Verification items for the finished model (mm, model axes). A direction names the side the tool comes from. Coordinates: 2 decimals unless noted, no trailing zeros. Order: outer loops, then holes, each group sorted by start corner. A loop starts at its lowest first (then second) coordinate and runs counter-clockwise, first axis right, second up.
Q1. Thickness scan on line 1 (X direction, y = 3, z = 6); line 2 (X direction, y = -8, z = 3.75); line 3 (X direction, y = -3, z = 0.5). Record the ranges inside material, lowest first.
Q2. Cross-section at D-D, the plane z = 1.25. Record the boundary of the cut face in (x, y), and give its area (3 significant figures).
Q3. Cross-section at B-B, the plane x = 0. Record the boundary of the cut face in (y, z) (3 decimals).
Q4. Depth check by flat-ended pin: P1, Ø10, axis at x = 2, y = -6, coming from the +Z side (3 decimals); P2, Ø1, axis at y = 10.5, z = 5.5, coming from the +X side; P3, Ø4.5, axis at x = -12.97, z = 4.76, coming from the +Y side; P4, Ø3, axis at x = -11.5, z = 4, coming from the +Y side. Enter the tip coordinate at first touch or a pass-through.
Q5. Draft check along Y on faces 1 (the flat face through (10, -12, 0)), 2 (the flat face through (26, 5.5, 7)), 3 (the flat face through (21, -1.5, 5)). Enter one of: pulls with the +Y half, pulls with the -Y half, needs draft (parallel to the pull), parting line crosses it, or undercut.
Q6. Cross-section at A-A, the plane y = -12.5. Record the boundary of the cut face in (x, z) (1 decimal), and give its area (3 significant figures).
Q7. Cross-section at C-C, the plane y = 10.5. Record the boundary of the cut face in (x, z) (3 decimals), and give its area (3 significant figures).
Q8. Set-up check for faces 4 (the flat face through (21, 1.5, 5)), 5 (the cylindrical face through (21.731, 3.472, 5.716)), 6 (the cylindrical face through (-14.572, -15.061, 5.991)): record each of +Z, -Z, +X, -X, +Y, -Y from which the full face is reachable in a straight line by a thin tool's end or side.
from build123d import *

# Parameters (mm, degrees)
BOSS_EXTRUDE1_DEPTH        = 9.525
F_10_CLEARANCE_HOLE1_D     = 4.9784
F_10_CLEARANCE_HOLE1_DEPTH = 4
F_10_CLEARANCE_HOLE1_TIP   = 1.495662253
F_10_32_TAPPED_HOLE1_D     = 4.0386
F_10_32_TAPPED_HOLE2_D     = 4.0386
F_10_32_TAPPED_HOLE2_DEPTH = 7
F_10_32_TAPPED_HOLE2_TIP   = 1.213317848


with BuildPart() as part:
    # Sketch1 → Boss-Extrude1 (new body)
    with BuildSketch(Plane.XY):
        with BuildLine():
            ThreePointArc((14.221111068, -1.5), (-14.3, 0), (14.221111068, 1.5))
            Line((14.221111068, 1.5), (28.530488985, 1.5))
            Line((28.530488985, 1.5), (28.530488985, 5.5))
            Line((28.530488985, 5.5), (19.530488985, 5.5))
            ThreePointArc((19.530488985, 5.5), (17.886036082, 5.990861772), (16.779715889, 7.302816901))
            ThreePointArc((16.779715889, 7.302816901), (-3.729691625, 17.915897979), (-18.3, 0))
            Line((-18.3, 0), (-18.3, -18.61))
            Line((-18.3, -18.61), (28.530488985, -18.61))
            Line((28.530488985, -18.61), (28.530488985, -1.5))
            Line((28.530488985, -1.5), (14.221111068, -1.5))
        make_face()
    extrude(amount=BOSS_EXTRUDE1_DEPTH)

    # #10 Clearance Hole1
    with Locations(Plane(origin=(0, 5.5, 0), x_dir=(1, 0, 0), z_dir=(0, 1, 0))):
        with Locations((24.030488985, -4.7625)):
            Hole(F_10_CLEARANCE_HOLE1_D / 2, depth=F_10_CLEARANCE_HOLE1_DEPTH)
            with Locations((0, 0, -(F_10_CLEARANCE_HOLE1_DEPTH + F_10_CLEARANCE_HOLE1_TIP / 2))):  # 118° drill point
                Cone(0, F_10_CLEARANCE_HOLE1_D / 2, F_10_CLEARANCE_HOLE1_TIP, mode=Mode.SUBTRACT)

    # #10-32 Tapped Hole1 (through all)
    with Locations(Plane(origin=(0, -1.5, 0), x_dir=(1, 0, 0), z_dir=(0, 1, 0))):
        with Locations((24.030488985, -4.7625)):
            Hole(F_10_32_TAPPED_HOLE1_D / 2)

    # #10-32 Tapped Hole2
    with Locations(Plane(origin=(0, -18.61, 0), x_dir=(-1, 0, 0), z_dir=(0, -1, 0))):
        with Locations((12.969511015, -4.7625)):
            Hole(F_10_32_TAPPED_HOLE2_D / 2, depth=F_10_32_TAPPED_HOLE2_DEPTH)
            with Locations((0, 0, -(F_10_32_TAPPED_HOLE2_DEPTH + F_10_32_TAPPED_HOLE2_TIP / 2))):  # 118° drill point
                Cone(0, F_10_32_TAPPED_HOLE2_D / 2, F_10_32_TAPPED_HOLE2_TIP, mode=Mode.SUBTRACT)


solid = part.part
Check values:
1. line 1: x = -18.05 to -13.98, 13.98 to 21.87, 26.19 to 28.53
1. line 2: x = -18.3 to -11.85, 11.85 to 22.28, 25.78 to 28.53
1. line 3: x = -18.3 to -13.98, 13.98 to 28.53
2. outline: (-18.3, -18.61) - (28.53, -18.61) - (28.53, -1.5) - (14.22, -1.5) arc R14.3 cw (long way) to (14.22, 1.5) - (28.53, 1.5) - (28.53, 5.5) - (19.53, 5.5) arc R3 cw to (16.78, 7.3) arc R18.3 ccw to (-18.3, 0) - close
2. area: 771 mm2
3. outline: (-18.61, 0) - (-14.3, 0) - (-14.3, 9.525) - (-18.61, 9.525) - close; (14.3, 0) - (18.3, 0) - (18.3, 9.525) - (14.3, 9.525) - close
4. P1: passes through
4. P2: stops at x = 15.33
4. P3: stops at y = 14.83
4. P4: stops at y = 15.33
5. face 1: needs draft
5. face 2: pulls with the +Y half
5. face 3: undercut
6. outline: (-18.3, 0) - (-6.9, 0) - (-6.9, 9.5) - (-18.3, 9.5) - close; (6.9, 0) - (28.5, 0) - (28.5, 9.5) - (6.9, 9.5) - close; hole circle Ø4 at (-13, 4.8); hole circle Ø4 at (24, 4.8)
6. area: 288 mm2
7. outline: (-14.988, 0) - (-9.708, 0) - (-9.708, 9.525) - (-14.988, 9.525) - close; (9.708, 0) - (14.988, 0) - (14.988, 9.525) - (9.708, 9.525) - close
7. area: 101 mm2
8. face 4: +Z, -Z, +X
8. face 5: +Y
8. face 6: -Y
